CAD build for the part. Positions are in the model's coordinates, mm. A direction names the side the tool comes from. Round coordinates to 2 decimals unless told otherwise and drop trailing zeros. Order: outer loops, then holes, each group sorted by start corner. A loop starts at its lowest first (then second) coordinate and runs counter-clockwise, first axis right, second up. Notation, with made-up numbers: M 69,38.25 L 123,38.25 A9 ccw 123,46.25 Z; hole C 82,45 d1. An arc over 180 degrees is marked long. Answer as a JSON object with one key per item and string values.
```python
from build123d import *

# Parameters (mm, degrees)
EXTRUDE_1_DEPTH            = 14
SKETCH_2_W                 = 10
SKETCH_2_H                 = 3
SKETCH_2_W_2               = 3
SKETCH_2_H_2               = 19
CUT_EXTRUDE_1_DEPTH        = 15
SKETCH_3_W                 = 8.5
SKETCH_3_H                 = 3
SKETCH_3_W_2               = 18.5
CUT_EXTRUDE_3_DEPTH        = 8
HOLE_WIZARD_M31_AT_2_COUNT = 2
HOLE_WIZARD_M31_AT_2_PITCH = 22
HOLE_WIZARD_M31_AT_3_COUNT = 2
HOLE_WIZARD_M31_AT_3_PITCH = 11
CUT_EXTRUDE_4_REACH        = 13.5


with BuildPart() as part:
    # Эскиз1 → Бобышка-Вытянуть1 (new body)
    with BuildSketch(Plane.XY):
        Polygon((-1.5, 0), (-1.5, 22), (-20, 22), (-20, 25), (20, 25), (20, 22), (1.5, 22), (1.5, 0), align=None)
    extrude(amount=EXTRUDE_1_DEPTH)

    # Эскиз2 → Вырез-Вытянуть1 (cut, through all)
    with BuildSketch(Plane.XY.offset(14)):
        with Locations((-15, 23.5)):
            Rectangle(SKETCH_2_W, SKETCH_2_H)
        with Locations((0, 9.5)):
            Rectangle(SKETCH_2_W_2, SKETCH_2_H_2)
    extrude(amount=-CUT_EXTRUDE_1_DEPTH, mode=Mode.SUBTRACT)

    # Эскиз3 → Вырез-Вытянуть3 (cut)
    with BuildSketch(Plane.XY.offset(14)):
        with Locations((-5.75, 23.5)):
            Rectangle(SKETCH_3_W, SKETCH_3_H)
        with Locations((10.75, 23.5)):
            Rectangle(SKETCH_3_W_2, SKETCH_3_H)
    extrude(amount=-CUT_EXTRUDE_3_DEPTH, mode=Mode.SUBTRACT)

    # Эскиз4 → Отверстие с зазором M31 (revolve, cut)
    with BuildSketch(Plane(origin=(-6.5, 22, 3), x_dir=(0, 0, -1), z_dir=(1, 0, 0))):
        Polygon((0, 0), (0, 3), (1.725, 3), (1.6, 2.875), (1.6, 0.125), (1.725, 0), align=None)
    hole_wizard_m31 = revolve(axis=Axis((-6.5, 15.65, 3), (0, 1, 0)), mode=Mode.SUBTRACT)

    # Отверстие с зазором M31 at 2: Отверстие с зазором M31 ×2
    with Locations(*[(i * HOLE_WIZARD_M31_AT_2_PITCH, 0, 0) for i in range(1, HOLE_WIZARD_M31_AT_2_COUNT)]):
        add(hole_wizard_m31, mode=Mode.SUBTRACT)

    # Отверстие с зазором M31 at 3: Отверстие с зазором M31 ×2
    with Locations(*[(i * HOLE_WIZARD_M31_AT_3_PITCH, 0, 0) for i in range(1, HOLE_WIZARD_M31_AT_3_COUNT)]):
        add(hole_wizard_m31, mode=Mode.SUBTRACT)

    # Эскиз6 → Вырез-Вытянуть4 (cut, up to next)
    with BuildSketch(Plane(origin=(1.5, 0, 0), x_dir=(0, 0, -1), z_dir=(1, 0, 0)), mode=Mode.PRIVATE) as cut_extrude_4_sk1:
        with BuildLine():
            Line((-11.35, 23.65), (-9.65, 23.65))
            ThreePointArc((-9.65, 23.65), (-8, 22), (-9.65, 20.35))
            Line((-9.65, 20.35), (-11.35, 20.35))
            ThreePointArc((-11.35, 20.35), (-13, 22), (-11.35, 23.65))
        make_face()
    cut_extrude_4_tool1 = extrude(cut_extrude_4_sk1.sketch, amount=-CUT_EXTRUDE_4_REACH, mode=Mode.PRIVATE) & part.part
    add(cut_extrude_4_tool1.solids().sort_by_distance((1.5, 22, 10.5))[0], mode=Mode.SUBTRACT)


solid = part.part
```
Item 1: Wall check: line 1 along X through (y, z) = (23.4, 3); line 2 along Z through (x, y) = (4.5, 23.4); line 3 along X through (y, z) = (22.9, 2.5). Give the ranges that are in metal, low to high. Write a range as [from, to].
Worked answers:
{"line 1": "x = [-10, -8.1], [-4.9, 2.9], [6.1, 13.9], [17.1, 20]", "line 2": "z = [0, 1.4], [4.6, 6]", "line 3": "x = [-10, -8.02], [-4.98, 2.98], [6.02, 13.98], [17.02, 20]"}
Item 2: Saw through at D-D on y = 21.2. List the corners of the cut face in (x, z).
Worked answers:
{"outline": "M -1.5,0 L 1.5,0 L 1.5,8.21 L -1.5,8.21 Z; M -1.5,12.79 L 1.5,12.79 L 1.5,14 L -1.5,14 Z"}
Item 3: Drop flat-ended pins along their axis: pin 1 Ø2.5 at (x, y) = (-7, 23.5) entering from +Z; pin 2 Ø4 at (x, z) = (-6.5, 3) entering from -Y; pin 3 Ø1.5 at (y, z) = (21, 7.5) entering from +X. Give the stop position or say it passes through.
Worked answers:
{"pin 1": "stops at z = 6", "pin 2": "stops at y = 22", "pin 3": "stops at x = 1.5"}
Item 4: Saw through at C-C on y = 23.3. List the corners of the cut face in (x, z).
Worked answers:
{"outline": "M -10,0 L 20,0 L 20,6 L 1.5,6 L 1.5,8.63 L -1.5,8.63 L -1.5,6 L -10,6 Z; M -1.5,12.37 L 1.5,12.37 L 1.5,14 L -1.5,14 Z; hole C -6.5,3 d3.2; hole C 4.5,3 d3.2; hole C 15.5,3 d3.2"}
Item 5: 3-axis set-ups, long thin cutter, end or side, ignore diameter. For faces 1 (the flat face through (11, 24, 6)), 2 (the cylindrical face through (0, 22, 8)), 3 (the flat face through (-6, 24, 6)), 4 (the flat face through (-4.7, 22, 2.3)): which of +Z, -Z, +X, -X, +Y, -Y reach the whole face in a straight line?
Worked answers:
{"face 1": "+Z, +X, +Y, -Y", "face 2": "+X, -X", "face 3": "+Z, -X, +Y, -Y", "face 4": "+Z, -Z, -X, -Y"}
Item 6: Saw through at A-A on x = 15.5. List the corners of the cut face in (y, z) (3 decimals), and give its area (3 significant figures).
Worked answers:
{"outline": "M 22,0 L 25,0 L 25,1.275 L 24.875,1.4 L 22.125,1.4 L 22,1.275 Z; M 22,4.725 L 22.125,4.6 L 24.875,4.6 L 25,4.725 L 25,6 L 22,6 Z", "area": "8.37 mm2"}
Item 7: Saw through at B-B on z = 10.25. List the corners of the cut face in (x, y), and give its area (3 significant figures).
Worked answers:
{"outline": "M -1.5,19 L 1.5,19 L 1.5,20.35 L -1.5,20.35 Z; M -1.5,23.65 L 1.5,23.65 L 1.5,25 L -1.5,25 Z", "area": "8.10 mm2"}
Item 8: Two-plate mould, pull along Y, no slides. Class faces 5 (the flat face through (5, 25, 5)), 6 (the cylindrical face through (13.914, 23.481, 3.208)), 7 (the flat face through (0, 23.65, 11)), 8 (the flat face through (0, 19, 7)): released by +Y, released by -Y, zero draft, split by the parting line, or undercut.
Worked answers:
{"face 5": "released by +Y", "face 6": "zero draft", "face 7": "undercut", "face 8": "released by -Y"}
